Autodesk Fusion 360 part; units mm, degrees
sketch "Sketch1" plane through (0, 0, 0) normal (0, 0, 1) x (1, 0, 0)
  line L0 (0, 0) -> (127, 0)
  line L1 (127, 0) -> (127, 68.58)
  line L2 (127, 68.58) -> (0, 68.58)
  line L3 (0, 68.58) -> (0, 0)
  line L4 (0, 0) -> (0, 34.29)
  line L5 (0, 34.29) -> (12.7, 34.29)
  line L6 (101.6, 0) -> (101.6, 63.5)
  line L7 (101.6, 63.5) -> (12.7, 63.5)
  line L8 (12.7, 63.5) -> (12.7, 0)
  line L9 (101.6, 5.08) -> (12.7, 5.08)
  dimension "d1" = 127
  dimension "d2" = 68.58
  dimension "d3" = 34.29
  dimension "d4" = 12.7
  dimension "d6" = 63.5
extrude "Extrude1" add sketch "Sketch1" against normal blind 22.86 contours L0 L3 L4 L5 L8 | L0 L6 L8 L9 | L0 L1 L2 L3 L5 L6 L7 L8
sketch "Sketch2" plane through (0, 0, 0) normal (-1, 0, 0) x (0, -1, 0)
  line L0 (0, 0) -> (-68.58, 0)
  line L1 (-68.58, 0) -> (-68.58, -22.86)
  line L2 (-68.58, -22.86) -> (0, -22.86)
  line L3 (0, -22.86) -> (0, 0)
  line L4 (-68.58, -22.86) -> (-68.58, -20.32)
  line L5 (-27.94, -20.32) -> (-27.94, -6.35)
  line L6 (-27.94, -6.35) -> (-48.26, -6.35)
  line L7 (-48.26, -6.35) -> (-48.26, -20.32)
  line L8 (-48.26, -20.32) -> (-27.94, -20.32)
  dimension "d12" = 13.97
extrude "Extrude2" cut sketch "Sketch2" against normal blind 5.08 contours L5 L6 L7 L8
sketch "Sketch3" plane through (101.6, 0, 0) normal (-1, 0, 0) x (0, -1, 0)
  line L0 (-5.08, 0) -> (-63.5, 0)
  line L1 (-63.5, 0) -> (-63.5, -22.86)
  line L2 (-63.5, -22.86) -> (-5.08, -22.86)
  line L3 (-5.08, -22.86) -> (-5.08, 0)
  line L4 (-63.5, -22.86) -> (-63.5, -1.27)
  line L5 (-63.5, -1.27) -> (-5.08, -1.27)
  line L6 (-5.08, -22.86) -> (-5.08, -1.27)
  line L7 (-63.5, -22.86) -> (-5.08, -22.86)
extrude "Extrude3" cut sketch "Sketch3" against normal blind 22.86 contours L1 L2 L3 L4 L5 L6 L7
sketch "Sketch4" plane through (12.7, 0, 0) normal (1, 0, 0) x (0, 1, 0)
  line L0 (63.5, 0) -> (5.08, 0)
  line L1 (5.08, 0) -> (5.08, -22.86)
  line L2 (5.08, -22.86) -> (63.5, -22.86)
  line L3 (63.5, -22.86) -> (63.5, 0)
  line L4 (5.08, -22.86) -> (5.08, -0.762)
  line L5 (5.08, -0.762) -> (63.5, -0.762)
  line L6 (63.5, -22.86) -> (63.5, -0.762)
  line L7 (63.5, -22.86) -> (5.08, -22.86)
extrude "Extrude4" cut sketch "Sketch4" against normal blind 10.16 contours L1 L2 L3 L4 L5 L6 L7
sketch "Sketch5" plane through (0, 63.5, 0) normal (0, -1, 0) x (1, 0, 0)
  line L0 (101.6, 0) -> (12.7, 0)
  line L1 (12.7, 0) -> (12.7, -0.762)
  line L2 (12.7, -0.762) -> (2.54, -0.762)
  line L3 (2.54, -0.762) -> (2.54, -22.86)
  line L4 (2.54, -22.86) -> (124.46, -22.86)
  line L5 (124.46, -22.86) -> (124.46, -1.27)
  line L6 (124.46, -1.27) -> (101.6, -1.27)
  line L7 (101.6, -1.27) -> (101.6, 0)
  line L8 (2.54, -0.762) -> (124.46, -1.27)
  line L9 (124.46, -22.86) -> (2.54, -22.86)
  line L10 (2.54, -0.762) -> (2.54, -21.3653)
extrude "Extrude5" cut sketch "Sketch5" against normal blind 3.81 contours L3 L4 L5 L6 L7 L8 L9 L10
sketch "Sketch6" plane through (0, 5.08, 0) normal (0, 1, 0) x (-1, 0, 0)
  line L0 (-12.7, 0) -> (-101.6, 0)
  line L1 (-101.6, 0) -> (-101.6, -1.27)
  line L2 (-101.6, -1.27) -> (-124.46, -1.27)
  line L3 (-124.46, -1.27) -> (-124.46, -22.86)
  line L4 (-124.46, -22.86) -> (-2.54, -22.86)
  line L5 (-2.54, -22.86) -> (-2.54, -0.762)
  line L6 (-2.54, -0.762) -> (-12.7, -0.762)
  line L7 (-12.7, -0.762) -> (-12.7, 0)
  line L8 (-124.46, -1.27) -> (-2.54, -0.762)
  line L9 (-2.54, -22.86) -> (-124.46, -22.86)
  line L10 (-124.46, -1.27) -> (-124.46, -22.86)
extrude "Extrude6" cut sketch "Sketch6" against normal blind 3.81 contours L1 L2 L3 L4 L5 L8 L9 L10
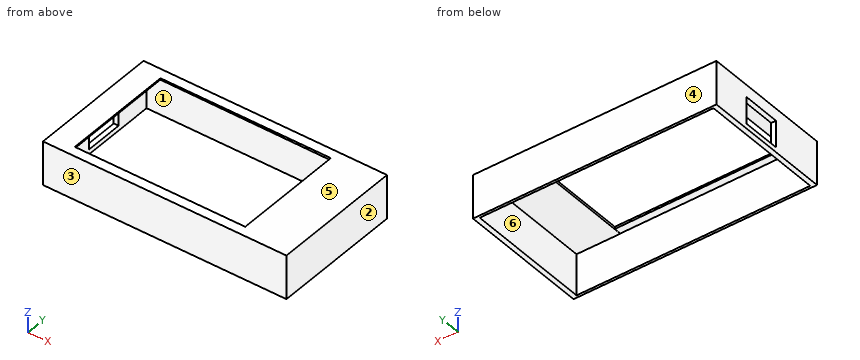
Verification items for the finished model (mm, model axes). Face numbers are marked on the shaded views. A direction names the side the tool comes from. Give positions to 0.01 mm unless a question says otherwise; leave off trailing zeros. Write each loop counter-clockwise with the first axis right and the second up, starting at its lowest first coordinate (ties: lowest second). Pieces come first, ordered by that corner, then holes.
(1) Access from +Z, -Z, +X, -X, +Y, -Y to the whole of each face (thin tool, end or side, straight path). Record for the marked faces 1 and 2.
(2) Cross-section at D-D (x = 103). Enter the section's corners in (y, z).
(3) Cross-section at A-A (y = 59). Enter the section's corners in (x, z), plus the area to 3 significant figures.
(4) Gauge pin test, flat ends, axial feed: pin 1 (5 mm diameter, centred on y = 49.5, z = -15, fed in from -X); pin 2 (7 mm diameter, centred on x = 108.5, y = 19, fed in from -Z); pin 3 (11 mm diameter, centred on x = 10, y = 41, fed in from -Z). Record the tip position at first contact, or that the pin passes through.
(5) Material ranges on line 1 (X direction, y = 52, z = -6.5); line 2 (Y direction, x = 80, z = -4.5); line 3 (Z direction, x = 117, y = 24), recorded low to high.
(6) Cross-section at B-B (x = 76). Enter the section's corners in (y, z).
(7) Mould release check, pull along Y, two halves, no side actions. Record for the marked faces 3, 4, 5 and 6: +Y half, -Y half, draft (parallel to the pull), parting line (faces both ways), or undercut.
(8) Cross-section at C-C (z = -12.5). Enter the section's corners in (x, y).
Worked out:
1. face 1: -Z
1. face 2: +Z, -Z, +X, +Y, -Y
2. outline: (0, -22.86) - (1.27, -22.86) - (1.27, -1.27) - (67.31, -1.27) - (67.31, -22.86) - (68.58, -22.86) - (68.58, 0) - (0, 0) - close
3. outline: (0, -22.86) - (2.54, -22.86) - (2.54, -0.76) - (12.7, -0.76) - (12.7, 0) - (0, 0) - close; (101.6, -1.27) - (124.46, -1.27) - (124.46, -22.86) - (127, -22.86) - (127, 0) - (101.6, 0) - close
3. area: 153 mm2
4. pin 1: stops at x = 0
4. pin 2: stops at z = -1.27
4. pin 3: stops at z = -0.76
5. line 1: x = 0 to 2.54, 124.46 to 127
5. line 2: y = 0 to 1.27, 67.31 to 68.58
5. line 3: z = -1.27 to 0
6. outline: (0, -22.86) - (1.27, -22.86) - (1.27, -1.07) - (5.08, -1.07) - (5.08, 0) - (0, 0) - close; (63.5, -1.07) - (67.31, -1.07) - (67.31, -22.86) - (68.58, -22.86) - (68.58, 0) - (63.5, 0) - close
7. face 3: -Y half
7. face 4: +Y half
7. face 5: draft
7. face 6: undercut
8. outline: (0, 0) - (127, 0) - (127, 68.58) - (0, 68.58) - (0, 48.26) - (2.54, 48.26) - (2.54, 67.31) - (124.46, 67.31) - (124.46, 1.27) - (2.54, 1.27) - (2.54, 27.94) - (0, 27.94) - close
